Answer from the drawing. Dimensions are ordinates in mm from the lowest x, y and z of the part. Coordinates: 2 decimals unless noted, no trailing zeros. Order: outer loops, then holes, each group sorted by start corner. A loop starts at its lowest first (then second) coordinate and runs counter-clockwise, first axis right, second up. Notation, with made-up numbers: (32.25, 51) -> (59.25, 51) arc R21 cw to (59.25, 68) -> close; hole circle Ø8 at (-30.75, -36.5). An arc over 180 degrees is marked (long way). Answer in a Markdown table with one row per item.
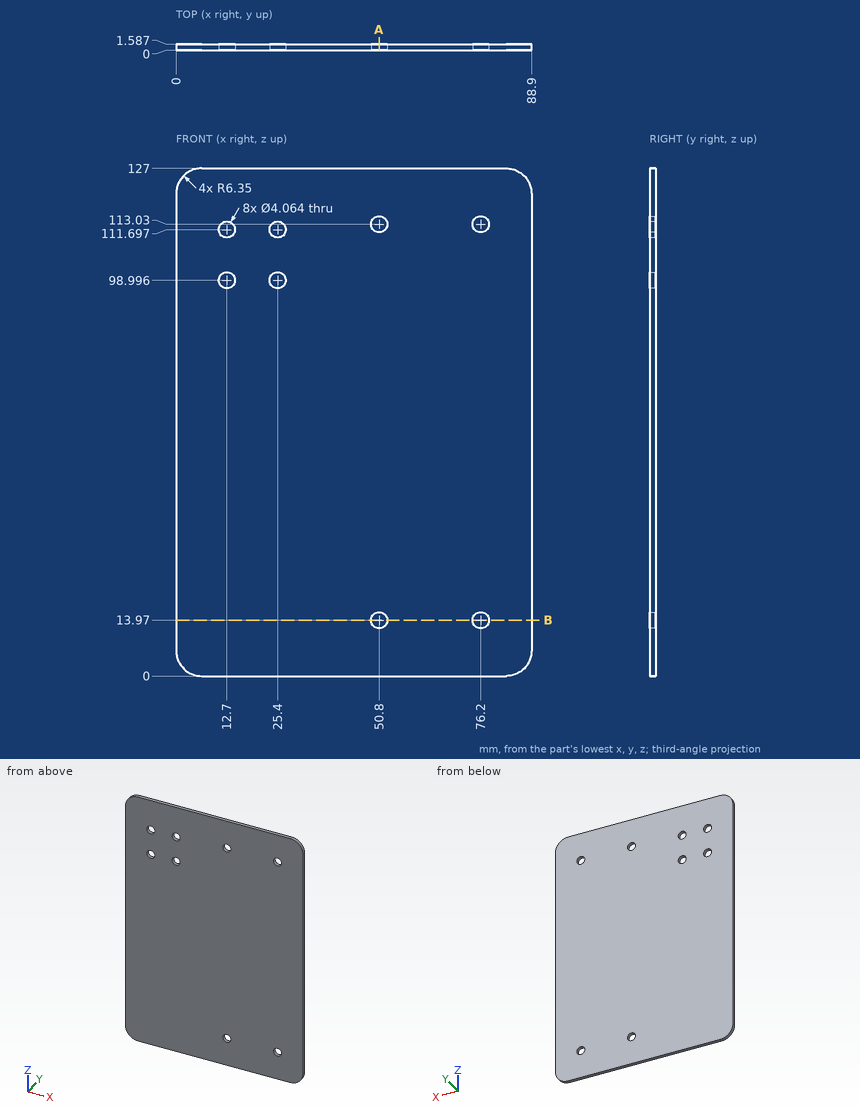
Q1. The part is cut by section A-A (x = 50.8). Write down the section's boundary in (y, z).
Outcome:
| item | result |
|---|---|
| outline | (0, 0) -> (1.59, 0) -> (1.59, 11.94) -> (0, 11.94) -> close; (0, 16) -> (1.59, 16) -> (1.59, 111) -> (0, 111) -> close; (0, 115.06) -> (1.59, 115.06) -> (1.59, 127) -> (0, 127) -> close |
Q2. Consider line 1 (X direction, y = 0.95, z = 13.97); line 2 (Z direction, x = 49.5, y = 0.75); line 3 (Z direction, x = 12, y = 0.4) (1 decimal). Determine where each line is inside the solid, lowest interval first.
Outcome:
| item | result |
|---|---|
| line 1 | 0 to 48.77, 52.83 to 74.17, 78.23 to 88.9 |
| line 2 | 0 to 12.41, 15.53 to 111.47, 114.59 to 127 |
| line 3 | 0 to 97.1, 100.9 to 109.8, 113.6 to 127 |
Q3. The part is cut by section B-B (z = 13.97). Write down the section's boundary in (x, y).
Outcome:
| item | result |
|---|---|
| outline | (0, 0) -> (48.77, 0) -> (48.77, 1.59) -> (0, 1.59) -> close; (52.83, 0) -> (74.17, 0) -> (74.17, 1.59) -> (52.83, 1.59) -> close; (78.23, 0) -> (88.9, 0) -> (88.9, 1.59) -> (78.23, 1.59) -> close |
